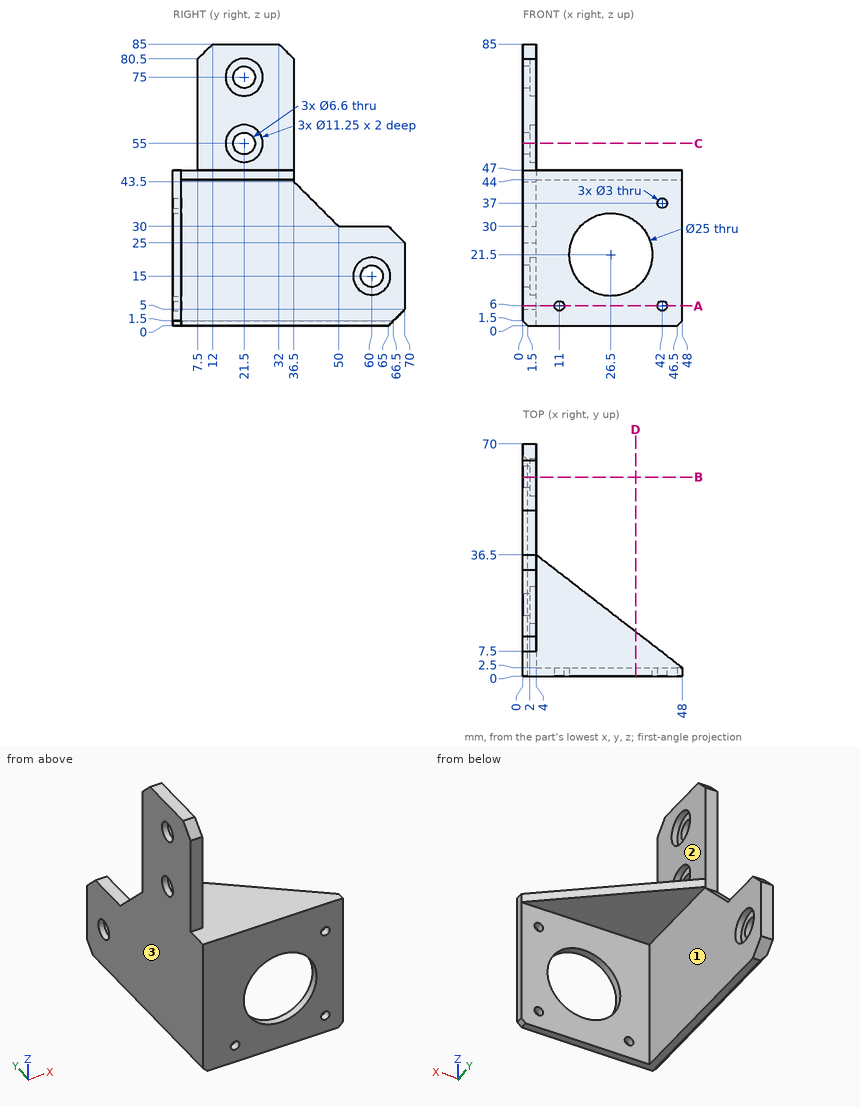
Answer from the drawing. Dimensions are ordinates in mm from the lowest x, y and z of the part. A direction names the side the tool comes from. Coordinates: 2 decimals unless noted, no trailing zeros. Order: outer loops, then holes, each group sorted by start corner. A loop starts at its lowest first (then second) coordinate and runs counter-clockwise, first axis right, second up. Notation, with made-up numbers: (-8.75, 50.5) - (13.25, 50.5) arc R13 ccw to (13.25, 57.5) - close; hole circle Ø1 at (68, 52.5). An arc over 180 degrees is marked (long way). Put each result on its own line as item: value. Start each with the question number.
1) For the marked faces 1, 2 and 3, determine the directions among +Z, -Z, +X, -X, +Y, -Y from which every point of the face is accessible in a straight line to the end or side of a thin tool.
2) Find the intervals of material crossed by line 1 (Z direction, x = 3.1, y = 21.5) (3 decimals); line 2 (Z direction, x = 26.5, y = 1.4); line 3 (X direction, y = 28, z = 7), in increasing order. Write a range as from..to.
3) Find section C-C (z = 55). Give the vertices of the cut face in (x, y) (3 decimals).
4) Find section A-A (z = 6). Give the vertices of the cut face in (x, y).
5) Find section B-B (y = 60). Give the vertices of the cut face in (x, z) (3 decimals), plus the area to 3 significant figures.
6) Flat-ended cylindrical pins translate along their axes: pin 1 (3 mm diameter, centred on y = 25.5, z = 59, fed in from +X); pin 2 (4 mm diameter, centred on x = 17.5, y = 14, fed in from -Z); pin 3 (5 mm diameter, centred on x = 42, z = 6, fed in from +Y). Find the tip coordinate at first contact, or state that the pin passes through.
7) Find section D-D (x = 34). Give the vertices of the cut face in (y, z).
Results list:
1. face 1: -Z, +X, +Y
1. face 2: +Z, +X, +Y, -Y
1. face 3: +Z, -Z, -X, +Y, -Y
2. line 1: z = 0..49.375, 60.625..69.375, 80.625..85
2. line 2: z = 0..9, 34..47
2. line 3: x = 0..4
3. outline: (0, 7.5) - (4, 7.5) - (4, 15.875) - (2, 15.875) - (2, 18.2) - (0, 18.2) - close; (0, 24.8) - (2, 24.8) - (2, 27.125) - (4, 27.125) - (4, 36.5) - (0, 36.5) - close
4. outline: (0, 0) - (9.5, 0) - (9.5, 2.5) - (4, 2.5) - (4, 70) - (0, 70) - close; (12.5, 0) - (40.5, 0) - (40.5, 2.5) - (12.5, 2.5) - close; (43.5, 0) - (48, 0) - (48, 2.5) - (43.5, 2.5) - close
5. outline: (0, 1.5) - (1.5, 0) - (4, 0) - (4, 9.375) - (2, 9.375) - (2, 11.7) - (0, 11.7) - close; (0, 18.3) - (2, 18.3) - (2, 20.625) - (4, 20.625) - (4, 30) - (0, 30) - close
5. area: 83.2 mm^2
6. pin 1: stops at x = 4
6. pin 2: stops at z = 44
6. pin 3: stops at y = 2.5
7. outline: (0, 0) - (2.5, 0) - (2.5, 11.5) - (0, 11.5) - close; (0, 31.5) - (2.5, 31.5) - (2.5, 44) - (13.32, 44) - (13.32, 47) - (0, 47) - close
